Here's how the part is built. I have some questions about the finished solid (model axes, mm). A direction names the side the tool comes from. Round coordinates to 2 decimals unless told otherwise and drop trailing zeros. Write each loop counter-clockwise with the first axis right and the second up, starting at its lowest first coordinate (ties: lowest second). Pieces come first, ordered by that corner, then holes. Notation, with made-up numbers: (-38.75, -31.5) - (13.25, -31.5) arc R23 cw to (13.25, -20.5) - close; hole circle Ø3 at (40.5, -29). An arc over 180 degrees is marked (long way). Write item = value, one per line. Start each with the question number.
Item 1: Thinking about a two-plate mould opening in X: for faces 6 (the face through (17.202, -68, 11)), 7 (the face through (-0.798, 29, 6)), 8 (the face through (-8, 9.788, 6)), which applies, pulls with the +X half, pulls with the -X half, needs draft (parallel to the pull), parting line crosses it, or undercut?
Item 2: For P1, Ø2, axis at x = -7.5, y = 29, coming from the +Z side; P2, Ø5, axis at x = 67, z = 6.5, coming from the +Y side; P3, Ø8, axis at x = 4, z = 13, coming from the -Y side; P4, Ø7.5, axis at y = -18, z = 5, coming from the -X side, each with a flat end and sliding along its axis, tell me the tip position at first contact or that it passes through.
Item 3: If I drill on line 1 along Y through (x, z) = (70.5, 9.5); line 2 along X through (y, z) = (-73, 10.25); line 3 along X through (y, z) = (18, 7), over which ranges is the centre line in solid material (lowest first)? Write a range as [from, to].
Item 4: Which directions (+Z, -Z, +X, -X, +Y, -Y) give clear straight access to the entire face, cutting with the end or side of a thin tool? Please do faces 1 (the face through (-0.798, -68, 11)), 2 (the face through (-15, -51, 14.5)), 3 (the face through (-0.798, -2, 6)), 4 (the face through (-8, 32.788, 6)), 5 (the face through (-0.798, -17, 6)).
Item 5: If we section it at A-A (y = -33.5): Please give me the cut outline in (x, z).
Item 6: If we section it at B-B (z = 7): Give the number of separate pieces and of enclosed holes in the cut face, and give its area (3 significant figures).
Item 7: If we section it at C-C (x = -5): Please give me the cut outline in (y, z).
Item 8: If we section it at D-D (y = -67.5): Please give me the cut outline in (x, z).
```python
from build123d import *

# Parameters (mm, degrees)
SKETCH_1_W      = 119
SKETCH_1_H      = 117.5
SKETCH_1_R      = 1.75
EXTRUDE_1_DEPTH = 1.5
SKETCH_2_W      = 15
SKETCH_2_H      = 12
EXTRUDE_2_DEPTH = 11.5
SKETCH_4_W      = 40
SKETCH_4_H      = 35.5
EXTRUDE_3_DEPTH = 28
SKETCH_5_W      = 5
SKETCH_5_H      = 17
EXTRUDE_4_DEPTH = 12
SKETCH_6_W      = 16
SKETCH_6_H      = 10
EXTRUDE_5_DEPTH = 13
SKETCH_7_W      = 18
SKETCH_7_H      = 22
EXTRUDE_6_DEPTH = 19
SKETCH_8_W      = 15
SKETCH_8_H      = 7
EXTRUDE_7_DEPTH = 9
SKETCH_9_W      = 16
SKETCH_9_H      = 10
EXTRUDE_9_DEPTH = 13


with BuildPart() as part:
    # Эскиз1 → Бобышка-Вытянуть1 (new body)
    with BuildSketch(Plane.XY):
        with Locations((32.702043262, -23.462126246)):
            Rectangle(SKETCH_1_W, SKETCH_1_H)
        with Locations((-22.297956738, 30.287873754)):
            Circle(SKETCH_1_R, mode=Mode.SUBTRACT)
        with Locations((87.702043262, 30.287873754)):
            Circle(SKETCH_1_R, mode=Mode.SUBTRACT)
        with Locations((87.702043262, -77.212126246)):
            Circle(SKETCH_1_R, mode=Mode.SUBTRACT)
        with Locations((-22.297956738, -77.212126246)):
            Circle(SKETCH_1_R, mode=Mode.SUBTRACT)
    extrude(amount=EXTRUDE_1_DEPTH)

    # Эскиз2 → Бобышка-Вытянуть2 (add)
    with BuildSketch(Plane.XY.offset(1.5)):
        with Locations((87.702043262, -6.712126246)):
            Rectangle(SKETCH_2_W, SKETCH_2_H)
    extrude(amount=EXTRUDE_2_DEPTH)

    # Эскиз4 → Бобышка-Вытянуть3 (add)
    with BuildSketch(Plane.XY.offset(1.5)):
        with Locations((66.202043262, -39.462126246)):
            Rectangle(SKETCH_4_W, SKETCH_4_H)
    extrude(amount=EXTRUDE_3_DEPTH)

    # Эскиз5 → Бобышка-Вытянуть4 (add)
    with BuildSketch(Plane.XY.offset(1.5)):
        with Locations((87.702043262, 15.287873754)):
            Rectangle(SKETCH_5_W, SKETCH_5_H)
        with Locations((78.702043262, 15.287873754)):
            Rectangle(SKETCH_5_W, SKETCH_5_H)
        with Locations((69.702043262, 15.287873754)):
            Rectangle(SKETCH_5_W, SKETCH_5_H)
        with Locations((60.702043262, 15.287873754)):
            Rectangle(SKETCH_5_W, SKETCH_5_H)
    extrude(amount=EXTRUDE_4_DEPTH)

    # Эскиз6 → Бобышка-Вытянуть5 (add)
    with BuildSketch(Plane.XY.offset(1.5)):
        with Locations((53.202043262, -69.212126246)):
            Rectangle(SKETCH_6_W, SKETCH_6_H)
        with Locations((74.202043262, -69.212126246)):
            Rectangle(SKETCH_6_W, SKETCH_6_H)
    extrude(amount=EXTRUDE_5_DEPTH)

    # Эскиз7 → Бобышка-Вытянуть6 (add)
    with BuildSketch(Plane.XY.offset(1.5)):
        with Locations((31.202043262, -67.712126246)):
            Rectangle(SKETCH_7_W, SKETCH_7_H)
        with Locations((8.202043262, -67.712126246)):
            Rectangle(SKETCH_7_W, SKETCH_7_H)
    extrude(amount=EXTRUDE_6_DEPTH)

    # Эскиз8 → Бобышка-Вытянуть7 (add)
    with BuildSketch(Plane.XY.offset(1.5)):
        with Locations((-8.297956738, 13.287873754)):
            Rectangle(SKETCH_8_W, SKETCH_8_H)
        with Locations((-8.297956738, -1.712126246)):
            Rectangle(SKETCH_8_W, SKETCH_8_H)
        with Locations((-8.297956738, -16.712126246)):
            Rectangle(SKETCH_8_W, SKETCH_8_H)
        with Locations((-8.297956738, -31.712126246)):
            Rectangle(SKETCH_8_W, SKETCH_8_H)
        with Locations((-8.297956738, 29.287873754)):
            Rectangle(SKETCH_8_W, SKETCH_8_H)
    extrude(amount=EXTRUDE_7_DEPTH)

    # Эскиз9 → Бобышка-Вытянуть9 (add)
    with BuildSketch(Plane.XY.offset(1.5)):
        with Locations((-14.797956738, -51.212126246)):
            Rectangle(SKETCH_9_W, SKETCH_9_H)
        with Locations((-14.797956738, -65.212126246)):
            Rectangle(SKETCH_9_W, SKETCH_9_H)
    extrude(amount=EXTRUDE_9_DEPTH)


solid = part.part
```
Reply:
q1.face_6 = undercut
q1.face_7 = pulls with the +X half
q1.face_8 = needs draft
q2.P1 = 10.5
q2.P2 = 23.79
q2.P3 = -78.71
q2.P4 = -26.8
q3.line_1 = [-74.21, -64.21], [-57.21, -21.71], [6.79, 23.79]
q3.line_2 = [-0.8, 17.2], [22.2, 40.2], [45.2, 61.2], [66.2, 82.2]
q3.line_3 = [58.2, 63.2], [67.2, 72.2], [76.2, 81.2], [85.2, 90.2]
q4.face_1 = +Z, -Y
q4.face_2 = +Z, -X, +Y, -Y
q4.face_3 = +Z, +Y
q4.face_4 = +Z, +X, -X, +Y
q4.face_5 = +Z, +X, +Y
q5.outline = (-26.8, 0) - (92.2, 0) - (92.2, 1.5) - (86.2, 1.5) - (86.2, 29.5) - (46.2, 29.5) - (46.2, 1.5) - (-0.8, 1.5) - (-0.8, 10.5) - (-15.8, 10.5) - (-15.8, 1.5) - (-26.8, 1.5) - close
q6.separate_pieces = 17
q6.enclosed_holes = 0
q6.area = 3,900 mm2
q7.outline = (-82.21, 0) - (35.29, 0) - (35.29, 1.5) - (32.79, 1.5) - (32.79, 10.5) - (25.79, 10.5) - (25.79, 1.5) - (16.79, 1.5) - (16.79, 10.5) - (9.79, 10.5) - (9.79, 1.5) - (1.79, 1.5) - (1.79, 10.5) - (-5.21, 10.5) - (-5.21, 1.5) - (-13.21, 1.5) - (-13.21, 10.5) - (-20.21, 10.5) - (-20.21, 1.5) - (-28.21, 1.5) - (-28.21, 10.5) - (-35.21, 10.5) - (-35.21, 1.5) - (-82.21, 1.5) - close
q8.outline = (-26.8, 0) - (92.2, 0) - (92.2, 1.5) - (82.2, 1.5) - (82.2, 14.5) - (66.2, 14.5) - (66.2, 1.5) - (61.2, 1.5) - (61.2, 14.5) - (45.2, 14.5) - (45.2, 1.5) - (40.2, 1.5) - (40.2, 20.5) - (22.2, 20.5) - (22.2, 1.5) - (17.2, 1.5) - (17.2, 20.5) - (-0.8, 20.5) - (-0.8, 1.5) - (-6.8, 1.5) - (-6.8, 14.5) - (-22.8, 14.5) - (-22.8, 1.5) - (-26.8, 1.5) - close
